Source: CAD feature listing. Evaluate the final solid. Frame: model axes, mm. Give positions to 0.01 mm unless a question says otherwise; leave off trailing zeros. Loops run counter-clockwise (first coordinate to the right, second up) from the corner with the lowest first, then second, coordinate; pieces in that order, holes last. Notation, with made-up numbers: M -23,17.25 L 25,17.25 A13 cw 25,38.25 Z; hole C 66,-21 d2. An arc over 180 degrees is marked long. Put each result on its own line as item: value.
from build123d import *

# Parameters (mm, degrees)
SKETCH1_R               = 55
BOSS_EXTRUDE1_DEPTH     = 3
SKETCH2_W               = 70
SKETCH2_H               = 100
BOSS_EXTRUDE2_DEPTH     = 3
SKETCH4_R               = 46
CUT_EXTRUDE2_DEPTH      = 1
CUT_EXTRUDE2_DEPTH_BACK = 4
CUT_EXTRUDE5_START      = -4
CUT_EXTRUDE5_DEPTH      = 5
CUT_EXTRUDE3_START      = -4
SKETCH5_R               = 2.25
CUT_EXTRUDE3_DEPTH      = 5
CIRPATTERN1_COUNT       = 12
CUT_EXTRUDE4_START      = -4
SKETCH6_R               = 3.25
CUT_EXTRUDE4_DEPTH      = 5
LPATTERN1_COUNT         = 3
LPATTERN1_PITCH         = 20


with BuildPart() as part:
    # Sketch1 → Boss-Extrude1 (new body)
    with BuildSketch(Plane(origin=(0, 0, 0), x_dir=(1, 0, 0), z_dir=(0, 1, 0))):
        Circle(SKETCH1_R)
    extrude(amount=BOSS_EXTRUDE1_DEPTH)

    # Sketch2 → Boss-Extrude2 (add)
    with BuildSketch(Plane(origin=(0, 0, 0), x_dir=(1, 0, 0), z_dir=(0, 1, 0))):
        with Locations((0, 92.426406871)):
            Rectangle(SKETCH2_W, SKETCH2_H)
    extrude(amount=BOSS_EXTRUDE2_DEPTH)

    # Sketch4 → Cut-Extrude2 (cut, two sides)
    with BuildSketch(Plane(origin=(0, 3, 0), x_dir=(1, 0, 0), z_dir=(0, 1, 0))) as cut_extrude2_sk:
        Circle(SKETCH4_R)
    extrude(amount=CUT_EXTRUDE2_DEPTH, mode=Mode.SUBTRACT)
    extrude(cut_extrude2_sk.sketch, amount=-CUT_EXTRUDE2_DEPTH_BACK, mode=Mode.SUBTRACT)

    # Sketch7 → Cut-Extrude5 (cut)
    with BuildSketch(Plane(origin=(0, 3, 0), x_dir=(1, 0, 0), z_dir=(0, 1, 0)).offset(CUT_EXTRUDE5_START)):
        with BuildLine():
            Line((0, 0), (0, -55))
            ThreePointArc((0, -55), (-24.969477486, -49.00535883), (-44.495934691, -32.328188876))
            Line((-44.495934691, -32.328188876), (0, 0))
        make_face()
    cut_extrude5 = extrude(amount=CUT_EXTRUDE5_DEPTH, mode=Mode.SUBTRACT)

    # Mirror1: Cut-Extrude5 across plane
    add(cut_extrude5.mirror(Plane(origin=(0, 0, 0), x_dir=(0, 0, 1), z_dir=(1, 0, 0))), mode=Mode.SUBTRACT)

    # Sketch5 → Cut-Extrude3 (cut)
    with BuildSketch(Plane(origin=(0, 3, 0), x_dir=(1, 0, 0), z_dir=(0, 1, 0)).offset(CUT_EXTRUDE3_START)):
        with Locations((0, 51)):
            Circle(SKETCH5_R)
    cut_extrude3 = extrude(amount=CUT_EXTRUDE3_DEPTH, mode=Mode.SUBTRACT)

    # CirPattern1: Cut-Extrude3 ×12 about axis
    cirpattern1_axis = Axis((0, 0, 0), (0, 1, 0))
    for i in range(1, CIRPATTERN1_COUNT):
        add(cut_extrude3.rotate(cirpattern1_axis, i * 360 / CIRPATTERN1_COUNT), mode=Mode.SUBTRACT)

    # Sketch6 → Cut-Extrude4 (cut)
    with BuildSketch(Plane(origin=(0, 3, 0), x_dir=(1, 0, 0), z_dir=(0, 1, 0)).offset(CUT_EXTRUDE4_START)):
        with Locations((15, 122.426406871)):
            Circle(SKETCH6_R)
        with Locations((-15, 122.426406871)):
            Circle(SKETCH6_R)
    cut_extrude4 = extrude(amount=CUT_EXTRUDE4_DEPTH, mode=Mode.SUBTRACT)

    # LPattern1: Cut-Extrude4 ×3
    with Locations(*[(0, 0, i * LPATTERN1_PITCH) for i in range(1, LPATTERN1_COUNT)]):
        add(cut_extrude4, mode=Mode.SUBTRACT)


solid = part.part
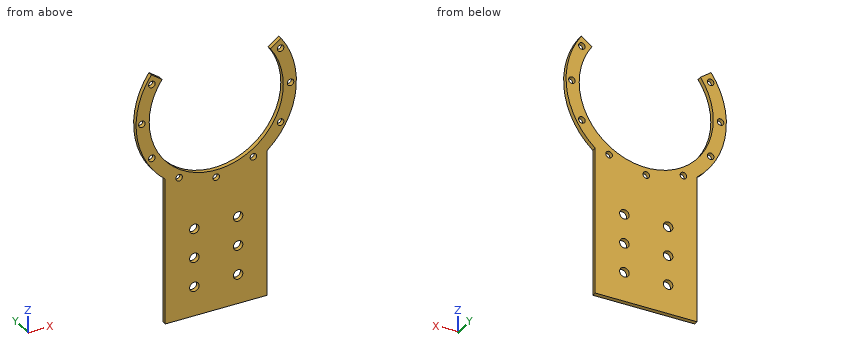
1. Section query A-A (z = 0). Output: boundary loops of the cut face in (x, y).
Found:
outline: M -55,0 L -53.25,0 L -53.25,3 L -55,3 Z; M -48.75,0 L -46,0 L -46,3 L -48.75,3 Z; M 46,0 L 48.75,0 L 48.75,3 L 46,3 Z; M 53.25,0 L 55,0 L 55,3 L 53.25,3 Z
2. Contact query for flat-ended pins moving along their axis: P1, Ø5, axis at x = -15, z = -82.43, coming from the +Y side; P2, Ø1.5, axis at y = 2, z = -84.5, coming from the -X side. Output: stop coordinate, or through.
Found:
P1: through
P2: x = -35
3. Section query D-D (y = 1.5). State how many separate pieces and enclosed holes the cut face has, plus the area to 3 significant figures.
Found:
separate pieces: 1
enclosed holes: 15
area: 8,060 mm^2
4. Material intervals for line 1 (Z direction, x = -15, y = 0.7); line 2 (X direction, y = 1.4, z = -85); line 3 (Z direction, x = -19, y = 0.4), sorted ascending. Write a range as from..to.
Found:
line 1: -142.43..-125.68, -119.18..-105.68, -99.18..-85.68, -79.18..-43.49
line 2: -35..-16.98, -13.02..13.02, 16.98..35
line 3: -142.43..-41.89
5. Section query B-B (x = 15). Output: boundary loops of the cut face in (y, z).
Found:
outline: M 0,-142.43 L 3,-142.43 L 3,-125.68 L 0,-125.68 Z; M 0,-119.18 L 3,-119.18 L 3,-105.68 L 0,-105.68 Z; M 0,-99.18 L 3,-99.18 L 3,-85.68 L 0,-85.68 Z; M 0,-79.18 L 3,-79.18 L 3,-43.49 L 0,-43.49 Z
6. Section query C-C (x = -25.5). Output: boundary loops of the cut face in (y, z).
Found:
outline: M 0,-142.43 L 3,-142.43 L 3,-46.42 L 0,-46.42 Z; M 0,-41.92 L 3,-41.92 L 3,-38.29 L 0,-38.29 Z
